Work out the finished part from the listing and answer in its coordinate system (mm). A direction names the side the tool comes from. Give positions to 0.01 mm unless a question says otherwise; leave off trailing zeros. Loops run counter-clockwise (first coordinate to the right, second up) from the corner with the lowest first, then second, coordinate; pieces in that order, holes last. Notation, with made-up numbers: (-36.5, 74.5) - (-19.5, 74.5) arc R18 ccw to (-19.5, 94.5) - close; hole circle Ø10 at (-23, -24). An arc over 180 degrees is marked (long way). One line per item, written item: value.
from build123d import *

# Parameters (mm, degrees)
SKETCH2_R          = 6
CUT_EXTRUDE1_DEPTH = 10
CUT_EXTRUDE2_DEPTH = 6


with BuildPart() as part:
    # Sketch1 → Revolve2 (revolve)
    with BuildSketch(Plane(origin=(0, 0, 0), x_dir=(1, 0, 0), z_dir=(0, 1, 0)), mode=Mode.PRIVATE) as revolve2_sk:
        with BuildLine():
            ThreePointArc((31, 42), (33.121320344, 42.878679656), (34, 45))
            Line((34, 45), (34, 72))
            Line((34, 72), (0, 72))
            Line((0, 72), (0, 78))
            Line((0, 78), (34, 78))
            Line((34, 78), (40, 72))
            Line((40, 72), (40, 42))
            Line((40, 42), (72, 42))
            Line((72, 42), (72, 32))
            Line((72, 32), (40, 32))
            Line((40, 32), (40, 4))
            Line((40, 4), (30, 0))
            Line((30, 0), (30, 42))
            Line((30, 42), (31, 42))
        make_face()
    revolve(revolve2_sk.sketch.rotate(Axis((0, 0, -115.849307743), (0, 0, 1)), 180), axis=Axis((0, 0, -115.849307743), (0, 0, 1)))

    # Sketch2 → Cut-Extrude1 (cut)
    with BuildSketch(Plane(origin=(0, 0, -42), x_dir=(-1, 0, 0), z_dir=(0, 0, -1))):
        with Locations((58, 0)):
            Circle(SKETCH2_R)
        with Locations((0, -58)):
            Circle(SKETCH2_R)
        with Locations((-58, 0)):
            Circle(SKETCH2_R)
        with Locations((0, 58)):
            Circle(SKETCH2_R)
    extrude(amount=-CUT_EXTRUDE1_DEPTH, mode=Mode.SUBTRACT)

    # Sketch3 → Cut-Extrude2 (cut)
    with BuildSketch(Plane(origin=(0, 0, -78), x_dir=(-1, 0, 0), z_dir=(0, 0, -1))):
        with BuildLine():
            Line((-6, 32), (6, 32))
            Line((6, 32), (6, 23.237900077))
            ThreePointArc((6, 23.237900077), (0, -24), (-6, 23.237900077))
            Line((-6, 23.237900077), (-6, 32))
        make_face()
    extrude(amount=-CUT_EXTRUDE2_DEPTH, mode=Mode.SUBTRACT)


solid = part.part
1. Find the intervals of material crossed by line 1 along Y through (x, z) = (0, -34); line 2 along Y through (x, z) = (0, -64); line 3 along Y through (x, z) = (0, -18), in increasing order.
Output:
line 1: y = -72 to -64, -52 to -30, 30 to 52, 64 to 72
line 2: y = -40 to -34, 34 to 40
line 3: y = -40 to -30, 30 to 40
2. Section D-D (x = 0) is taken. Count the separate pieces of the cut face and the enclosed holes in it, and give its area (3 significant figures).
Output:
separate pieces: 4
enclosed holes: 0
area: 1,670 mm²
3. The mould has two halves that part along Z. Classify faces 5 (the flat face through (6, 28, -75)), 6 (the flat face through (-7.1, -23.1, -72)), 7 (the flat face through (31, 31, -42)), 8 (the flat face through (-31, 31, -32)): released by +Z, released by -Z, zero draft, split by the parting line, or undercut.
Output:
face 5: zero draft
face 6: undercut
face 7: released by -Z
face 8: released by +Z
4. Section A-A (x = 58) is taken. Write down the section's boundary in (y, z).
Output:
outline: (-42.66, -42) - (-6, -42) - (-6, -32) - (-42.66, -32) - close; (6, -42) - (42.66, -42) - (42.66, -32) - (6, -32) - close
5. For faces 1 (the cylindrical face through (-52, 0, -37)), 2 (the cylindrical face through (39.96, -1.76, -56.79)), 3 (the cylindrical face through (39.96, -1.76, -17.8)), 4 (the flat face through (-28, -12, -42)), determine the directions among +Z, -Z, +X, -X, +Y, -Y from which every point of the face is accessible in a straight line to the end or side of a thin tool.
Output:
face 1: +Z, -Z
face 2: -Z
face 3: +Z
face 4: none
6. Flat-ended cylindrical pins translate along their axes: pin 1 Ø6.5 at (x, z) = (2.5, -75) entering from -Y; pin 2 Ø12 at (x, y) = (-53.5, 12.5) entering from +Z; pin 3 Ø8 at (x, z) = (11.5, -12) entering from -Y. Find the tip coordinate at first contact, or state that the pin passes through.
Output:
pin 1: stops at y = -39.98
pin 2: stops at z = -32
pin 3: stops at y = -39.29
7. Section C-C (z = -55) is taken. Write down the section's boundary in (x, y), and give its area (3 significant figures).
Output:
outline: circle Ø80 at (0, 0); hole circle Ø68 at (0, 0)
area: 1,390 mm²
